The model under review builds one solid part; all positions refer to its coordinate system, in mm. Face numbers are marked on the shaded views. A direction names the side the tool comes from. Round coordinates to 2 decimals unless told otherwise and drop trailing zeros. Loops run counter-clockwise (first coordinate to the right, second up) from the corner with the lowest first, then second, coordinate; pieces in that order, holes last. Notation, with made-up numbers: M 89.5,3 L 147.5,3 A21 cw 147.5,34 Z; hole C 54.5,-22.5 d4. An arc over 180 degrees is marked long. Use a Markdown table: item, result. Add a question column.
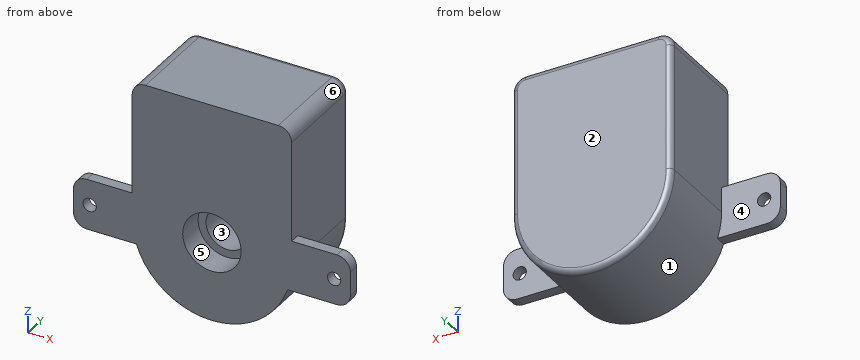
```python
from build123d import *

# Parameters (mm, degrees)
BOSS_EXTRUDE1_DEPTH = 18.3
SKETCH2_R           = 1.25
BOSS_EXTRUDE2_DEPTH = 2
FILLET1_R           = 2.5
SKETCH3_R           = 5.5
CUT_EXTRUDE2_DEPTH  = 5
SKETCH5_R           = 4
CUT_EXTRUDE3_DEPTH  = 15
FILLET2_R           = 1


with BuildPart() as part:
    # Sketch1 → Boss-Extrude1 (new body)
    with BuildSketch(Plane(origin=(0, 0, 0), x_dir=(1, 0, 0), z_dir=(0, 1, 0))):
        with BuildLine():
            Line((-15, 0), (-15, -26.1))
            Line((-15, -26.1), (15, -26.1))
            Line((15, -26.1), (15, 0))
            ThreePointArc((15, 0), (0, 15), (-15, 0))
        make_face()
    extrude(amount=BOSS_EXTRUDE1_DEPTH)

    # Sketch2 → Boss-Extrude2 (add)
    with BuildSketch(Plane(origin=(0, 0, 0), x_dir=(1, 0, 0), z_dir=(0, 1, 0))):
        with BuildLine():
            Line((23.55, -4.75), (-23.55, -4.75))
            ThreePointArc((-23.55, -4.75), (-25.317766953, -4.017766953), (-26.05, -2.25))
            Line((-26.05, -2.25), (-26.05, 2.25))
            ThreePointArc((-26.05, 2.25), (-25.317766953, 4.017766953), (-23.55, 4.75))
            Line((-23.55, 4.75), (23.55, 4.75))
            ThreePointArc((23.55, 4.75), (25.317766953, 4.017766953), (26.05, 2.25))
            Line((26.05, 2.25), (26.05, -2.25))
            ThreePointArc((26.05, -2.25), (25.317766953, -4.017766953), (23.55, -4.75))
        make_face()
        with Locations((-23, 0)):
            Circle(SKETCH2_R, mode=Mode.SUBTRACT)
        with Locations((23, 0)):
            Circle(SKETCH2_R, mode=Mode.SUBTRACT)
    extrude(amount=BOSS_EXTRUDE2_DEPTH)

    # Fillet1
    fillet1_edges = [part.edges().sort_by_distance(p)[0] for p in [
        (15, 9.15, 26.1),
        (-15, 9.15, 26.1),
    ]]
    fillet(fillet1_edges, radius=FILLET1_R)

    # Sketch3 → Cut-Extrude2 (cut)
    with BuildSketch(Plane(origin=(0, 0, 0), x_dir=(-1, 0, 0), z_dir=(0, -1, 0))):
        with Locations((0, 0.1)):
            Circle(SKETCH3_R)
    extrude(amount=-CUT_EXTRUDE2_DEPTH, mode=Mode.SUBTRACT)

    # Sketch5 → Cut-Extrude3 (cut)
    with BuildSketch(Plane(origin=(0, 0, 0), x_dir=(-1, 0, 0), z_dir=(0, -1, 0))):
        with Locations((0, 0.1)):
            Circle(SKETCH5_R)
    extrude(amount=-CUT_EXTRUDE3_DEPTH, mode=Mode.SUBTRACT)

    # Fillet2
    fillet2_edges = [part.edges().sort_by_distance(p)[0] for p in [
        (0, 18.3, -15),
        (0, 18.3, 26.1),
        (15, 18.3, 11.8),
        (14.267766953, 18.3, 25.367766953),
        (-14.267766953, 18.3, 25.367766953),
        (-15, 18.3, 11.8),
    ]]
    fillet(fillet2_edges, radius=FILLET2_R)


solid = part.part
```
(1) For the marked faces 1, 2 and 3, list the 3-axis set-ups (+Z, -Z, +X, -X, +Y, -Y) from which the entire face can be reached by the end or side of a thin tool; tool diameter is ignored.
(2) To check wall thickness, follow probe 1 along X at (y, z) = (0.9, 0); probe 2 along Z at (x, y) = (23, 0.5). State the ranges of each line that lie inside material, in increasing order.
(3) Consider section A-A, the plane y = 12. Give the boundary of the cut face in (x, z), then the cut area to 3 significant figures.
(4) Draft analysis for pull direction Z (two halves, no side actions). For the marked faces 4, 5 and 6, state which applies: released by +Z, released by -Z, zero draft, split by the parting line, or undercut.
(5) Consider section B-B, the plane x = 0. Give the boundary of the cut face in (y, z), then the cut area to 3 significant figures.
(6) Insertion check: pin 1 Ø3.5 at (x, z) = (1, 2.5) entering from -Y; pin 2 Ø1 at (x, y) = (-21, 1) entering from -Z; pin 3 Ø3 at (x, z) = (-18.5, 1) entering from +Y; pin 4 Ø8 at (x, y) = (-16, 6) entering from +Z. Each pin has a flat end and moves straight along its axis. Give the tip position at first contact, or say it passes through.
(7) Consider section C-C, the plane y = 3. Give the boundary of the cut face in (x, z), then the cut area to 3 significant figures.
(8) Consider section D-D, the plane x = -17. Give the boundary of the cut face in (y, z), then the cut area to 3 significant figures.
Found:
| question | item | result |
|---|---|---|
| 1 | face 1 | -Z, +Y |
| 1 | face 2 | +Z, -Z, +X, -X, +Y |
| 1 | face 3 | -Y |
| 2 | probe 1 | x = -26.05 to -24.25, -21.75 to -5.5, 5.5 to 21.75, 24.25 to 26.05 |
| 2 | probe 2 | z = -4.75 to -1.25, 1.25 to 4.75 |
| 3 | outline | M -15,0 A15 ccw 15,0 L 15,23.6 A2.5 ccw 12.5,26.1 L -12.5,26.1 A2.5 ccw -15,23.6 Z; hole C 0,-0.1 d8 |
| 3 | area | 1,080 mm^2 |
| 4 | face 4 | zero draft |
| 4 | face 5 | undercut |
| 4 | face 6 | released by +Z |
| 5 | outline | M 0,-15 L 17.3,-15 A1 ccw 18.3,-14 L 18.3,25.1 A1 ccw 17.3,26.1 L 0,26.1 L 0,5.4 L 5,5.4 L 5,3.9 L 15,3.9 L 15,-4.1 L 5,-4.1 L 5,-5.6 L 0,-5.6 Z |
| 5 | area | 617 mm^2 |
| 6 | pin 1 | stops at y = 5 |
| 6 | pin 2 | stops at z = -4.75 |
| 6 | pin 3 | stops at y = 2 |
| 6 | pin 4 | stops at z = 26.1 |
| 7 | outline | M -15,0 A15 ccw 15,0 L 15,23.6 A2.5 ccw 12.5,26.1 L -12.5,26.1 A2.5 ccw -15,23.6 Z; hole C 0,-0.1 d11 |
| 7 | area | 1,040 mm^2 |
| 8 | outline | M 0,-4.75 L 2,-4.75 L 2,4.75 L 0,4.75 Z |
| 8 | area | 19.0 mm^2 |
